from build123d import *

# Parameters (mm, degrees)
ESBO_O1_R                 = 9.327345029
RESSALTO_EXTRUS_O1_DEPTH  = 3
FILETE1_R                 = 10
ESBO_O2_R                 = 1
CORTE_EXTRUS_O1_DEPTH     = 123.545028697
FILETE3_R                 = 4
FILETE3_OF_ESPELHAR1_R    = 4
ESPELHAR2_OUTLINE_R       = 1
ESPELHAR2_DEPTH           = 3
ESBO_O4_R                 = 1.5
CORTE_EXTRUS_O3_DEPTH     = 123.545028697
ESPELHAR4_COPY_1_SKETCH_R = 1.5
ESPELHAR4_COPY_1_DEPTH    = 123.545028697
ESBO_O5_R                 = 1
CORTE_EXTRUS_O4_DEPTH     = 123.545028697


# Read off the part's stored shape, not the designer's step: Espelhar2
with BuildPart() as part:
    # Esboço1 → Ressalto-extrusão1 (new body)
    with BuildSketch(Plane(origin=(0, 0, 0), x_dir=(1, 0, 0), z_dir=(0, 1, 0))):
        with BuildLine():
            ThreePointArc((69.076751756, -72.307692308), (91.944752911, -39.321271752), (100, 0))
            ThreePointArc((100, 0), (91.944752911, 39.321271752), (69.076751756, 72.307692308))
            ThreePointArc((69.076751756, 72.307692308), (0, 60), (-69.076751756, 72.307692308))
            ThreePointArc((-69.076751756, 72.307692308), (-100, 0), (-69.076751756, -72.307692308))
            ThreePointArc((-69.076751756, -72.307692308), (0, -60), (69.076751756, -72.307692308))
        make_face()
        with Locations(Location((0, 0, 0), (0, 0, 270))):
            Circle(ESBO_O1_R, mode=Mode.SUBTRACT)
    extrude(amount=RESSALTO_EXTRUS_O1_DEPTH)

    # Filete1
    filete1_edges = [part.edges().sort_by_distance(p)[0] for p in [
        (-69.076751756, 1.5, -72.307692308),
        (69.076751756, 1.5, -72.307692308),
        (69.076751756, 1.5, 72.307692308),
        (-69.076751756, 1.5, 72.307692308),
    ]]
    fillet(filete1_edges, radius=FILETE1_R)

    # Esboço2 → Corte-extrusão1 (cut, through all)
    with BuildSketch(Plane(origin=(0, 3, 0), x_dir=(1, 0, 0), z_dir=(0, 1, 0))):
        with BuildLine():
            Line((58.172237404, 62.817121833), (81.047076875, 27.592957979))
            Line((81.047076875, 27.592957979), (87.41930694, 31.731132569))
            ThreePointArc((87.41930694, 31.731132569), (83.247103811, 41.459856573), (77.996361738, 50.651431921))
            ThreePointArc((77.996361738, 50.651431921), (71.735109934, 59.186772195), (64.544467469, 66.955296423))
            Line((64.544467469, 66.955296423), (58.172237404, 62.817121833))
        make_face()
        with Locations(Location((27.220325105, 30.793082034, 0), (0, 0, 270))):
            Circle(ESBO_O2_R)
        with Locations(Location((39.202383876, 12.342329539, 0), (0, 0, 270))):
            Circle(ESBO_O2_R)
        with Locations(Location((59.425274915, 51.707220979, 0), (0, 0, 270))):
            Circle(ESBO_O2_R)
        with Locations(Location((71.407333685, 33.256468484, 0), (0, 0, 270))):
            Circle(ESBO_O2_R)
    corte_extrus_o1 = extrude(amount=-CORTE_EXTRUS_O1_DEPTH, mode=Mode.SUBTRACT)

    # Filete3
    filete3_edges = [part.edges().sort_by_distance(p)[0] for p in [
        (87.41930694, 1.5, -31.731132569),
        (81.047076875, 1.5, -27.592957979),
        (58.172237404, 1.5, -62.817121833),
        (64.544467469, 1.5, -66.955296423),
    ]]
    fillet(filete3_edges, radius=FILETE3_R)

    # Espelhar1: Corte-extrusão1 across plane
    add(corte_extrus_o1.mirror(Plane(origin=(0, 0, 0), x_dir=(0, 0, 1), z_dir=(1, 0, 0))), mode=Mode.SUBTRACT)

    # Filete3 of Espelhar1
    filete3_of_espelhar1_edges = [part.edges().sort_by_distance(p)[0] for p in [
        (-87.41930694, 1.5, -31.731132569),
        (-81.047076875, 1.5, -27.592957979),
        (-58.172237404, 1.5, -62.817121833),
        (-64.544467469, 1.5, -66.955296423),
    ]]
    fillet(filete3_of_espelhar1_edges, radius=FILETE3_OF_ESPELHAR1_R)

    # Espelhar2 outline → Espelhar2 (cut)
    with BuildSketch(Plane(origin=(0, 0, 0), x_dir=(1, 0, 0), z_dir=(0, 1, 0))):
        with BuildLine():
            Line((-61.829947011, -65.192466226), (-61.526919676, -64.995677973))
            ThreePointArc((-61.526919676, -64.995677973), (-59.792885413, -62.472642464), (-60.350793544, -59.462439561))
            Line((-60.350793544, -59.462439561), (-78.868520735, -30.947640251))
            ThreePointArc((-78.868520735, -30.947640251), (-81.391556244, -29.213605988), (-84.401759147, -29.771514119))
            Line((-84.401759147, -29.771514119), (-84.704786482, -29.968302372))
            ThreePointArc((-84.704786482, -29.968302372), (-86.340974216, -32.119768464), (-86.235274402, -34.820646875))
            ThreePointArc((-86.235274402, -34.820646875), (-77.996362819, -50.651430256), (-66.88528981, -64.617010199))
            ThreePointArc((-66.88528981, -64.617010199), (-64.460906593, -65.812118002), (-61.829947011, -65.192466226))
        make_face()
        with BuildLine():
            ThreePointArc((61.829947011, -65.192466226), (64.460906593, -65.812118002), (66.88528981, -64.617010199))
            ThreePointArc((66.88528981, -64.617010199), (77.996362819, -50.651430256), (86.235274402, -34.820646875))
            ThreePointArc((86.235274402, -34.820646875), (86.340974216, -32.119768464), (84.704786482, -29.968302372))
            Line((84.704786482, -29.968302372), (84.401759147, -29.771514119))
            ThreePointArc((84.401759147, -29.771514119), (81.391556244, -29.213605988), (78.868520735, -30.947640251))
            Line((78.868520735, -30.947640251), (60.350793544, -59.462439561))
            ThreePointArc((60.350793544, -59.462439561), (59.792885413, -62.472642464), (61.526919676, -64.995677973))
            Line((61.526919676, -64.995677973), (61.829947011, -65.192466226))
        make_face()
        with Locations((-27.220325105, -30.793082034)):
            Circle(ESPELHAR2_OUTLINE_R)
        with Locations((-39.202383876, -12.342329539)):
            Circle(ESPELHAR2_OUTLINE_R)
        with Locations((-59.425274915, -51.707220979)):
            Circle(ESPELHAR2_OUTLINE_R)
        with Locations((-71.407333685, -33.256468484)):
            Circle(ESPELHAR2_OUTLINE_R)
        with Locations((27.220325105, -30.793082034)):
            Circle(ESPELHAR2_OUTLINE_R)
        with Locations((39.202383876, -12.342329539)):
            Circle(ESPELHAR2_OUTLINE_R)
        with Locations((59.425274915, -51.707220979)):
            Circle(ESPELHAR2_OUTLINE_R)
        with Locations((71.407333685, -33.256468484)):
            Circle(ESPELHAR2_OUTLINE_R)
    extrude(amount=ESPELHAR2_DEPTH, mode=Mode.SUBTRACT)

    # Esboço4 → Corte-extrusão3 (cut, through all)
    with BuildSketch(Plane(origin=(0, 3, 0), x_dir=(1, 0, 0), z_dir=(0, 1, 0))):
        with Locations(Location((-50, 55, 0), (0, 0, 270))):
            Circle(ESBO_O4_R)
    corte_extrus_o3 = extrude(amount=-CORTE_EXTRUS_O3_DEPTH, mode=Mode.SUBTRACT)

    # Espelhar3: Corte-extrusão3 across plane
    add(corte_extrus_o3.mirror(Plane(origin=(0, 0, 0), x_dir=(0, 0, 1), z_dir=(1, 0, 0))), mode=Mode.SUBTRACT)

    # Espelhar4: Corte-extrusão3 across plane
    add(corte_extrus_o3.mirror(Plane.XY), mode=Mode.SUBTRACT)

    # Espelhar4 copy 1 sketch → Espelhar4 copy 1 (cut, through all)
    with BuildSketch(Plane(origin=(0, 3, 0), x_dir=(-1, 0, 0), z_dir=(0, 1, 0))):
        with Locations(Location((-50, 55, 0), (0, 0, 270))):
            Circle(ESPELHAR4_COPY_1_SKETCH_R)
    extrude(amount=-ESPELHAR4_COPY_1_DEPTH, mode=Mode.SUBTRACT)

    # Esboço5 → Corte-extrusão4 (cut, through all)
    with BuildSketch(Plane(origin=(0, 3, 0), x_dir=(1, 0, 0), z_dir=(0, 1, 0))):
        with Locations(Location((23, 55, 0), (0, 0, 270))):
            Circle(ESBO_O5_R)
        with Locations(Location((23, 41, 0), (0, 0, 270))):
            Circle(ESBO_O5_R)
        with Locations(Location((-23, 55, 0), (0, 0, 90))):
            Circle(ESBO_O5_R)
        with Locations(Location((-23, 41, 0), (0, 0, 90))):
            Circle(ESBO_O5_R)
        with Locations(Location((-23, -41, 0), (0, 0, 270))):
            Circle(ESBO_O5_R)
        with Locations(Location((-23, -55, 0), (0, 0, 270))):
            Circle(ESBO_O5_R)
        with Locations(Location((23, -55, 0), (0, 0, 90))):
            Circle(ESBO_O5_R)
        with Locations(Location((23, -41, 0), (0, 0, 90))):
            Circle(ESBO_O5_R)
    extrude(amount=-CORTE_EXTRUS_O4_DEPTH, mode=Mode.SUBTRACT)


solid = part.part
Geometry check sheet. Reference: the model listing, model coordinates, mm. A direction names the side the tool comes from. Give positions to 0.01 mm unless a question says otherwise; leave off trailing zeros. Write each loop counter-clockwise with the first axis right and the second up, starting at its lowest first coordinate (ties: lowest second). Pieces come first, ordered by that corner, then holes.
1) Release check for a two-part mould opening along Z. For faces 1 (the face through (2.802, 1.479, 8.897)), 2 (the face through (-0.901, 1.479, 60.002)), 3 (the face through (-1, 3, -17)) record: released by +Z, released by -Z, zero draft, split by the parting line, or undercut.
Values follow:
face 1: undercut
face 2: released by +Z
face 3: zero draft
2) Set-up check for faces 4 (the face through (77.86, 1.48, 50.86)), 5 (the face through (-1, 0, -17)): record each of +Z, -Z, +X, -X, +Y, -Y from which the full face is reachable in a straight line by a thin tool's end or side.
Values follow:
face 4: +Y, -Y
face 5: +Z, -Z, +X, -X, -Y
3) Go/stop test with flat-tipped pins: pin 1 Ø1.5 at (x, y) = (-31.5, 1) entering from +Z; pin 2 Ø1.5 at (x, y) = (44.5, 0.5) entering from -Z; pin 3 Ø2.5 at (x, z) = (71.41, 33.26) entering from +Y. Record where each tip stops, or that it passes through.
Values follow:
pin 1: stops at z = 62.62
pin 2: stops at z = -65.19
pin 3: stops at y = 3
4) Cross-section at B-B (y = 0.85). Count the separate pieces of the cut face and the enclosed holes in it, plus the area to 3 significant figures.
Values follow:
separate pieces: 1
enclosed holes: 33
area: 22,000 mm2
5) Cross-section at A-A (z = -38). Record the boundary of the cut face in (x, y), plus the area to 3 significant figures.
Values follow:
outline: (-92.5, 0) - (-84.88, 0) - (-84.88, 3) - (-92.5, 3) - close; (-74.29, 0) - (74.29, 0) - (74.29, 3) - (-74.29, 3) - close; (84.88, 0) - (92.5, 0) - (92.5, 3) - (84.88, 3) - close
area: 491 mm2
6) Cross-section at C-C (x = -14). Record the boundary of the cut face in (y, z).
Values follow:
outline: (0, -60.49) - (3, -60.49) - (3, 60.49) - (0, 60.49) - close
7) Thickness scan on line 1 (X direction, y = 1.95, z = 47.5); line 2 (Z direction, x = -49, y = 0.35); line 3 (X direction, y = 1.5, z = -41). Record the ranges inside material, lowest first.
Values follow:
line 1: x = -88 to -79.95, -68.12 to 68.12, 79.95 to 88
line 2: z = -66.1 to -56.12, -53.88 to 53.88, 56.12 to 66.1
line 3: x = -91.21 to -83.47, -72.34 to -24, -22 to 22, 24 to 72.34, 83.47 to 91.21
